Design review of the part shown in the three views and the two pictorial views. Dimensions are in mm from the part's minimum x, y and z. A direction names the side the tool comes from. Give positions to 0.01 mm unless a question says otherwise; leave off trailing zeros. Order: outer loops, then holes, each group sorted by start corner. A loop starts at its lowest first (then second) coordinate and runs counter-clockwise, first axis right, second up.
Item 1: The part is to be moulded in two halves that separate along X. For the marked faces 1, 2, 3 and 4, say which applies: released by +X, released by -X, zero draft, split by the parting line, or undercut.
Item 2: Consider section C-C (z = 5). Give the boundary of the cut face in (x, y).
Item 3: For P1, Ø5, axis at x = 127, y = 15, coming from the -Z side; P2, Ø6, axis at x = 62.5, z = 10, coming from the -Y side; P3, Ø1.5, axis at y = 9, z = 12.5, coming from the -X side; P4, Ø3, axis at x = 114.5, z = 7, coming from the -Y side, all flat-tipped, find the tip position at first contact; note any pin that passes through.
Item 4: Consider section A-A (y = 15). Give the boundary of the cut face in (x, z), plus the area to 4 significant figures.
Item 5: Consider section D-D (x = 127). Give the boundary of the cut face in (y, z), plus the area to 3 significant figures.
Item 6: For probe 1 along X at (y, z) = (15.25, 13.5); probe 2 along Y at (x, z) = (127, 3); probe 3 along X at (y, z) = (16, 8), list the stretches that pass through material, from the lowest coordinate up.
Item 7: Machinability: for the marked faces 5 and 6, which of the approach directions +Z, -Z, +X, -X, +Y, -Y give a long, thin tool a straight path to every point of the face, cutting with its end or side? Answer none if there is none.
Item 8: Consider section B-B (x = 74). Give the boundary of the cut face in (y, z), plus the area to 3 significant figures.
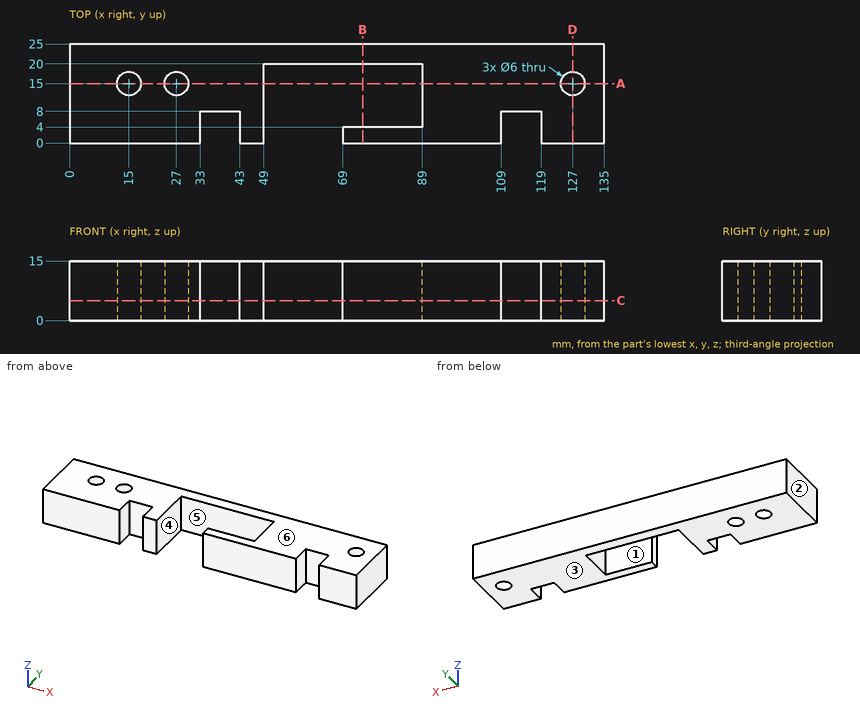
Resolved:
1. face 1: undercut
1. face 2: released by -X
1. face 3: zero draft
1. face 4: undercut
2. outline: (0, 0) - (33, 0) - (33, 8) - (43, 8) - (43, 0) - (49, 0) - (49, 20) - (89, 20) - (89, 4) - (69, 4) - (69, 0) - (109, 0) - (109, 8) - (119, 8) - (119, 0) - (135, 0) - (135, 25) - (0, 25) - close; hole circle Ø6 at (15, 15); hole circle Ø6 at (27, 15); hole circle Ø6 at (127, 15)
3. P1: passes through
3. P2: stops at y = 20
3. P3: stops at x = 0
3. P4: stops at y = 8
4. outline: (0, 0) - (12, 0) - (12, 15) - (0, 15) - close; (18, 0) - (24, 0) - (24, 15) - (18, 15) - close; (30, 0) - (49, 0) - (49, 15) - (30, 15) - close; (89, 0) - (124, 0) - (124, 15) - (89, 15) - close; (130, 0) - (135, 0) - (135, 15) - (130, 15) - close
4. area: 1,155 mm2
5. outline: (0, 0) - (12, 0) - (12, 15) - (0, 15) - close; (18, 0) - (25, 0) - (25, 15) - (18, 15) - close
5. area: 285 mm2
6. probe 1: x = 0 to 12.01, 17.99 to 24.01, 29.99 to 49, 89 to 124.01, 129.99 to 135
6. probe 2: y = 0 to 12, 18 to 25
6. probe 3: x = 0 to 12.17, 17.83 to 24.17, 29.83 to 49, 89 to 124.17, 129.83 to 135
7. face 5: +Z, -Z
7. face 6: +Z, +X, -X, +Y, -Y
8. outline: (0, 0) - (4, 0) - (4, 15) - (0, 15) - close; (20, 0) - (25, 0) - (25, 15) - (20, 15) - close
8. area: 135 mm2
